CAD build for the part. Positions are in the model's coordinates, mm. A direction names the side the tool comes from. Give positions to 0.01 mm unless a question says otherwise; leave off trailing zeros. Write each loop counter-clockwise with the first axis right and the second up, starting at its lowest first coordinate (ties: lowest second). Pieces come first, ordered by that corner, then holes. Notation, with made-up numbers: (8, -24) -> (60, -24) arc R36 cw to (60, 11) -> close; hole circle Ø7 at (-28.5, 28). An arc over 180 degrees is marked (long way). Answer as a JSON object with one key per item and string values.
```python
from build123d import *

# Parameters (mm, degrees)
F2_DEPTH = 41.3
F3_T     = -0.8
F4_SIZE  = 0.5


with BuildPart() as f2:
    # F1 (on Front) → F2 (new body)
    with BuildSketch(Plane.XZ):
        Polygon((0, 27), (0, 0), (25, 0), (30, 5), (30, 27), align=None)
    extrude(amount=-F2_DEPTH)

    # F3
    f3_openings = [f2.faces().sort_by_distance(p)[0] for p in [
        (14.791014, 0, 13.685475),
    ]]
    offset(amount=F3_T, openings=f3_openings)

    # F4
    f4_edges = [f2.edges().sort_by_distance(p)[0] for p in [
        (15, 0, 26.2),
        (29.2, 0, 15.765685),
        (26.934315, 0, 3.065685),
        (12.734315, 0, 0.8),
        (0.8, 0, 13.5),
    ]]
    chamfer(f4_edges, length=F4_SIZE)


solid = f2.part
```
1) Slice it at C-C (y = 33). List the corners of the cut face in (x, z).
Model answer:
{"outline": "(0, 0) -> (25, 0) -> (30, 5) -> (30, 27) -> (0, 27) -> close; hole (0.8, 0.8) -> (24.67, 0.8) -> (29.2, 5.33) -> (29.2, 26.2) -> (0.8, 26.2) -> close"}
2) Slice it at A-A (x = 19.75). List the corners of the cut face in (y, z), then the cut area to 4 significant figures.
Model answer:
{"outline": "(0, 0) -> (41.3, 0) -> (41.3, 27) -> (0, 27) -> (0, 26.7) -> (0.5, 26.2) -> (40.5, 26.2) -> (40.5, 0.8) -> (0.5, 0.8) -> (0, 0.3) -> close", "area": "86.15 mm2"}
3) Slice it at B-B (z = 6.5). List the corners of the cut face in (x, y).
Model answer:
{"outline": "(0, 0) -> (0.3, 0) -> (0.8, 0.5) -> (0.8, 40.5) -> (29.2, 40.5) -> (29.2, 0.5) -> (29.7, 0) -> (30, 0) -> (30, 41.3) -> (0, 41.3) -> close"}
4) Wall check: probe 1 along Z at (x, y) = (21, 9); probe 2 along X at (y, z) = (27, 9); probe 3 along Y at (x, z) = (5, 2.75). Give the ranges that are in metal, low to high.
Model answer:
{"probe 1": "z = 0 to 0.8, 26.2 to 27", "probe 2": "x = 0 to 0.8, 29.2 to 30", "probe 3": "y = 40.5 to 41.3"}
5) Mould opens along X. For faces 1 (the flat face through (30, 20, 16)), 2 (the flat face through (15, 40.5, 14)), 3 (the flat face through (15, 20, 27)) say: released by +X, released by -X, zero draft, split by the parting line, or undercut.
Model answer:
{"face 1": "released by +X", "face 2": "undercut", "face 3": "zero draft"}
6) Pin check, flat tip, straight feed: pin 1 (1 mm diameter, centred on x = 15, z = 22.5, fed in from -Y). Stop position of the tip, or through.
Model answer:
{"pin 1": "stops at y = 40.5"}
7) 3-axis set-ups, long thin cutter, end or side, ignore diameter. For faces 4 (the flat face through (26.9, 20.22, 3.03)), 5 (the flat face through (27, 20, 2)): which of +Z, -Z, +X, -X, +Y, -Y reach the whole face in a straight line?
Model answer:
{"face 4": "-Y", "face 5": "-Z, +X, +Y, -Y"}
